Geometry: see drawing. Coordinates: mm, zero at the bounding-box minimum. Give positions to 0.01 mm unless a question says otherwise; leave off trailing zeros. Write each loop counter-clockwise with the first axis right and the second up, starting at its lowest first coordinate (ties: lowest second). Pieces come first, ordered by that corner, then holes.
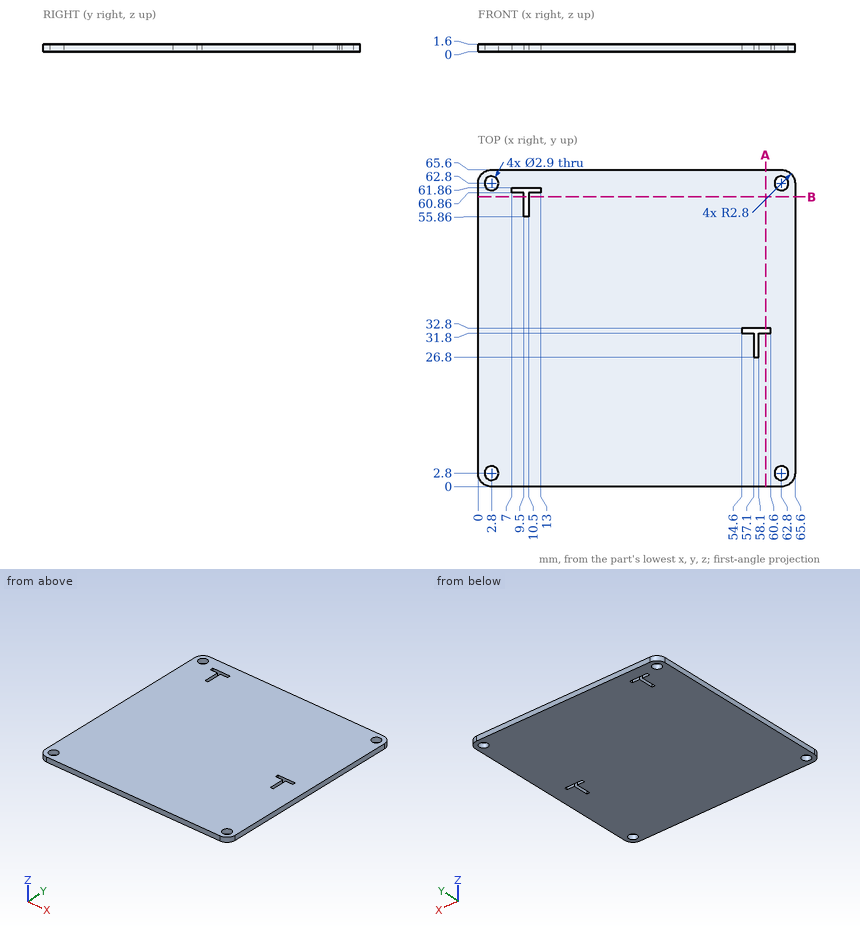
Q1. Pin query (flat end, axial travel): pin 1 (3.5 mm diameter, centred on x = 2.8, y = 62.8, fed in from -Z); pin 2 (1.7 mm diameter, centred on x = 2.8, y = 2.8, fed in from +Z). Return the tip coordinate at first contact, or that it passes through.
Q2. Section A-A, the plane x = 59.5. Return the cut outline in (y, z).
Q3. Material intervals for line 1 along Y through (x, z) = (2.8, 0.4); line 2 along X through (y, z) = (29.5, 1.3); line 3 along X through (y, z) = (63.5, 0.6), sorted ascending.
Q4. Section B-B, the plane y = 60. Return the cut outline in (x, z), then the cut area to 3 significant figures.
Solutions:
1. pin 1: stops at z = 0
1. pin 2: passes through
2. outline: (0, 0) - (31.8, 0) - (31.8, 1.6) - (0, 1.6) - close; (32.8, 0) - (65.6, 0) - (65.6, 1.6) - (32.8, 1.6) - close
3. line 1: y = 0 to 1.35, 4.25 to 61.35, 64.25 to 65.6
3. line 2: x = 0 to 57.1, 58.1 to 65.6
3. line 3: x = 0.09 to 1.53, 4.07 to 61.53, 64.07 to 65.51
4. outline: (0, 0) - (9.5, 0) - (9.5, 1.6) - (0, 1.6) - close; (10.5, 0) - (65.6, 0) - (65.6, 1.6) - (10.5, 1.6) - close
4. area: 103 mm2
